Geometry check sheet. Reference: drawing and pictorial views, mm from the part's lowest x, y, z. Coordinates: 2 decimals unless noted, no trailing zeros. Answer as a JSON object with one key per item and string values. Group by question number.
Q1. Release check for a two-part mould opening along Z. For the marked faces 1, 2 and 3 record: released by +Z, released by -Z, zero draft, split by the parting line, or undercut.
Q2. Scan lines: L1, parallel to Z at x = 11, y = 4.25 (1 decimal); L2, parallel to Z at x = 6.25, y = 5.75 (1 decimal); L3, parallel to X at y = 5.5, z = 11.25. Record each from-to range of solid material in increasing order.
Q3. Gauge pin test, flat ends, axial feed: pin 1 Ø6 at (x, y) = (6, 7) entering from -Z; pin 2 Ø6 at (x, z) = (9.5, 10.97) entering from +Y; pin 3 Ø1.5 at (y, z) = (7, 3) entering from +X (1 decimal). Record the tip position at first contact, or that the pin passes through.
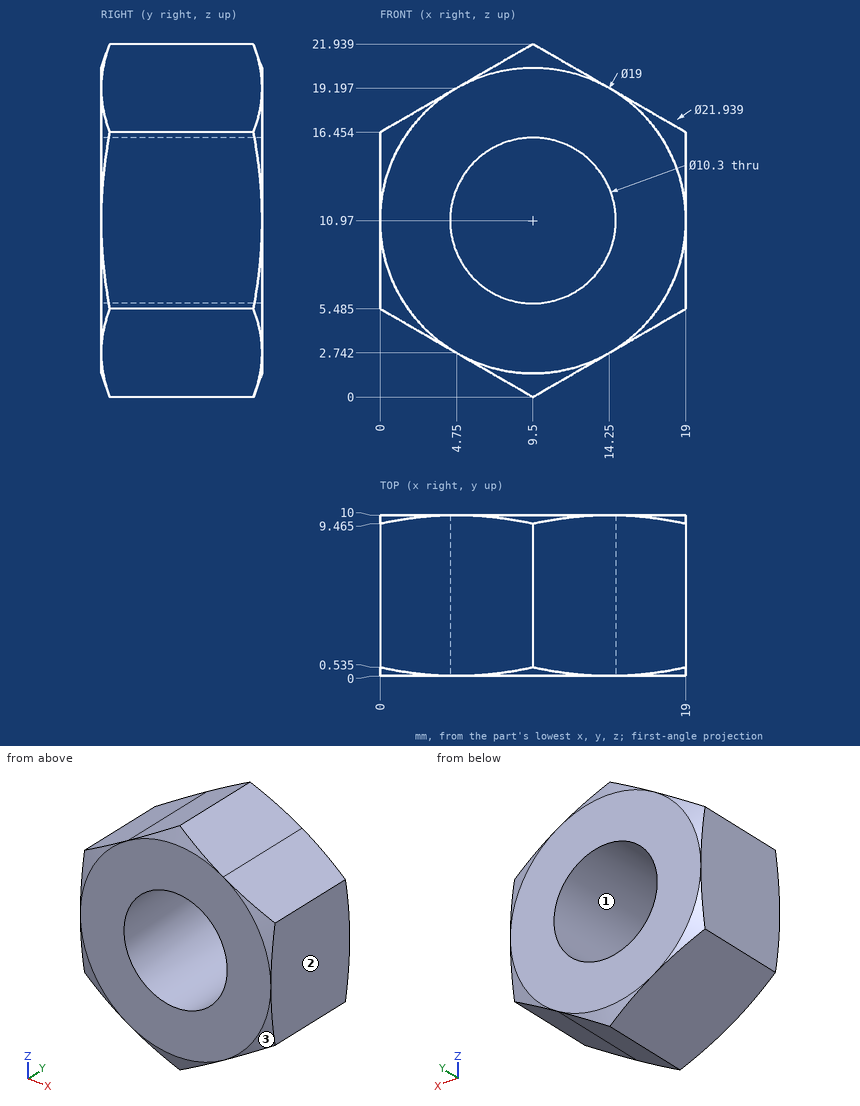
Computed values:
{
 "1": {"face 1": "undercut", "face 2": "zero draft", "face 3": "released by -Z"},
 "2": {"L1": "z = 0.9 to 6, 15.9 to 21.1", "L2": "z = 1.9 to 7, 15 to 20.1", "L3": "x = 0 to 4.36, 14.64 to 19"},
 "3": {"pin 1": "stops at z = 0.29", "pin 2": "passes through", "pin 3": "stops at x = 16"}
}
